from build123d import *

# Parameters (mm, degrees)
SKETCH1_W           = 40
SKETCH1_H           = 48.8
BOSS_EXTRUDE1_DEPTH = 1
SKETCH2_W           = 40
SKETCH2_H           = 48.8
SKETCH2_W_2         = 38
SKETCH2_H_2         = 35.8
BOSS_EXTRUDE2_DEPTH = 4
SKETCH3_W           = 20.5
SKETCH3_H           = 8
CUT_EXTRUDE1_DEPTH  = 6
BOSS_EXTRUDE3_REACH = 7
SKETCH4_W           = 6.5
SKETCH4_H           = 5
SKETCH5_W           = 7
SKETCH5_H           = 11
BOSS_EXTRUDE4_DEPTH = 2.8
SKETCH7_W           = 10
SKETCH7_H           = 4.5
BOSS_EXTRUDE5_DEPTH = 4


with BuildPart() as part:
    # Sketch1 → Boss-Extrude1 (new body)
    with BuildSketch(Plane(origin=(0, 0, 0), x_dir=(1, 0, 0), z_dir=(0, 1, 0))):
        Rectangle(SKETCH1_W, SKETCH1_H)
    extrude(amount=BOSS_EXTRUDE1_DEPTH)

    # Sketch2 → Boss-Extrude2 (add)
    with BuildSketch(Plane(origin=(0, 1, 0), x_dir=(1, 0, 0), z_dir=(0, 1, 0))):
        Rectangle(SKETCH2_W, SKETCH2_H)
        Rectangle(SKETCH2_W_2, SKETCH2_H_2, mode=Mode.SUBTRACT)
    extrude(amount=BOSS_EXTRUDE2_DEPTH)

    # Sketch3 → Cut-Extrude1 (cut, through all)
    with BuildSketch(Plane(origin=(0, 5, 0), x_dir=(1, 0, 0), z_dir=(0, 1, 0))):
        with Locations((0, -24.4)):
            Rectangle(SKETCH3_W, SKETCH3_H)
        with Locations((0, 24.4)):
            Rectangle(SKETCH3_W, SKETCH3_H)
    extrude(amount=-CUT_EXTRUDE1_DEPTH, mode=Mode.SUBTRACT)

    # Sketch4 → Boss-Extrude3 (add, up to next)
    with BuildSketch(Plane(origin=(0, 5, 0), x_dir=(1, 0, 0), z_dir=(0, 1, 0)), mode=Mode.PRIVATE) as boss_extrude3_sk1:
        with Locations((-15.75, -15.4)):
            Rectangle(SKETCH4_W, SKETCH4_H)
    boss_extrude3_tool1 = extrude(boss_extrude3_sk1.sketch, amount=-BOSS_EXTRUDE3_REACH, mode=Mode.PRIVATE) - part.part
    add(boss_extrude3_tool1.solids().sort_by_distance((-15.75, 5, 15.4))[0])
    # Sketch4 → Boss-Extrude3 (add, up to next)
    with BuildSketch(Plane(origin=(0, 5, 0), x_dir=(1, 0, 0), z_dir=(0, 1, 0)), mode=Mode.PRIVATE) as boss_extrude3_sk2:
        with Locations((-15.75, 15.4)):
            Rectangle(SKETCH4_W, SKETCH4_H)
    boss_extrude3_tool2 = extrude(boss_extrude3_sk2.sketch, amount=-BOSS_EXTRUDE3_REACH, mode=Mode.PRIVATE) - part.part
    add(boss_extrude3_tool2.solids().sort_by_distance((-15.75, 5, -15.4))[0])
    # Sketch4 → Boss-Extrude3 (add, up to next)
    with BuildSketch(Plane(origin=(0, 5, 0), x_dir=(1, 0, 0), z_dir=(0, 1, 0)), mode=Mode.PRIVATE) as boss_extrude3_sk3:
        Polygon((19, 17.9), (19, -17.9), (13.150842714, -17.9), (13.150842714, -12.9), (14, -12.9), (14, 12.9), (12.5, 12.9), (12.5, 17.9), align=None)
    boss_extrude3_tool3 = extrude(boss_extrude3_sk3.sketch, amount=-BOSS_EXTRUDE3_REACH, mode=Mode.PRIVATE) - part.part
    add(boss_extrude3_tool3.solids().sort_by_distance((16.307114, 5, -0.262731))[0])

    # Sketch5 → Boss-Extrude4 (add)
    with BuildSketch(Plane.XZ):
        with Locations((-16, -2.6)):
            Rectangle(SKETCH5_W, SKETCH5_H)
    extrude(amount=-BOSS_EXTRUDE4_DEPTH)

    # Sketch7 → Boss-Extrude5 (add)
    with BuildSketch(Plane.ZY.offset(20)):
        with Locations((7.9, 2.25)):
            Rectangle(SKETCH7_W, SKETCH7_H)
    extrude(amount=-BOSS_EXTRUDE5_DEPTH)


solid = part.part
Input: part model. Units: mm. Frame: model coordinates. A direction names the side the tool comes from. Give positions to 0.01 mm unless a question says otherwise; leave off trailing zeros. Order: outer loops, then holes, each group sorted by start corner. A loop starts at its lowest first (then second) coordinate and runs counter-clockwise, first axis right, second up. Notation, with made-up numbers: M 13.25,-25 L 66.25,-25 A23 ccw 66.25,-11 Z; hole C 66,2.25 d10. An arc over 180 degrees is marked long. Answer as a JSON object with one key per item and string values.
1. Cut plane D-D, the plane z = 6. Output: boundary loops of the cut face in (x, y), and give its area (3 significant figures).
Result sheet:
{"outline": "M -20,0 L 20,0 L 20,5 L 14,5 L 14,1 L -16,1 L -16,4.5 L -19,4.5 L -19,5 L -20,5 Z", "area": "78.5 mm²"}
2. Reachability of faces 4 (the flat face through (12.5, 3, -15)), 5 (the flat face through (0, 3, 20.4)), 6 (the flat face through (0, 3, -20.4)) from +Z, -Z, +X, -X, +Y, -Y: full face, straight path, thin tool, end or side. Return the list, or none.
Result sheet:
{"face 4": "+Y", "face 5": "+Z, +Y, -Y", "face 6": "-Z, +Y, -Y"}
3. Cut plane C-C, the plane z = -14. Output: boundary loops of the cut face in (x, y).
Result sheet:
{"outline": "M -20,0 L 20,0 L 20,5 L 12.5,5 L 12.5,1 L -12.5,1 L -12.5,5 L -20,5 Z"}
4. Pull-direction query (Z, two-part tool) for faces 1 (the flat face through (-16, 3, -12.9)), 2 (the flat face through (-15, 2, 24.4)), 3 (the flat face through (10.25, 3, -22)); classes: +Z half, -Z half, draft (parallel to the pull), parting line (faces both ways), or undercut.
Result sheet:
{"face 1": "undercut", "face 2": "+Z half", "face 3": "draft"}
5. Cut plane A-A, the plane y = 2.2. Output: boundary loops of the cut face in (x, z), and give its area (3 significant figures).
Result sheet:
{"outline": "M -20,-24.4 L -10.25,-24.4 L -10.25,-20.4 L 10.25,-20.4 L 10.25,-24.4 L 20,-24.4 L 20,24.4 L 10.25,24.4 L 10.25,20.4 L -10.25,20.4 L -10.25,24.4 L -20,24.4 Z; hole M -19,-12.9 L -12.5,-12.9 L -12.5,-17.9 L 12.5,-17.9 L 12.5,-12.9 L 14,-12.9 L 14,12.9 L 13.15,12.9 L 13.15,17.9 L -12.5,17.9 L -12.5,12.9 L -16,12.9 L -16,2.9 L -12.5,2.9 L -12.5,-8.1 L -19,-8.1 Z", "area": "785 mm²"}
6. First-contact query: P1, Ø7, axis at x = -14.5, z = -1.5, coming from the +Y side. Flat tip, straight axial feed; report the tip coordinate or a pass-through.
Result sheet:
{"P1": "y = 2.8"}
7. Ray query, line 1 (Z direction, x = -15.5, y = 2.9); line 2 (Z direction, x = 12, y = 4.3); line 3 (X direction, y = 2.65, z = -4). Return the intervals inside material, ascending. Write a range as [from, to].
Result sheet:
{"line 1": "[-24.4, -12.9], [12.9, 24.4]", "line 2": "[-24.4, -17.9], [17.9, 24.4]", "line 3": "[-20, -12.5], [14, 20]"}
8. Cut plane B-B, the plane x = 5. Output: boundary loops of the cut face in (y, z).
Result sheet:
{"outline": "M 0,-20.4 L 5,-20.4 L 5,-17.9 L 1,-17.9 L 1,17.9 L 5,17.9 L 5,20.4 L 0,20.4 Z"}
